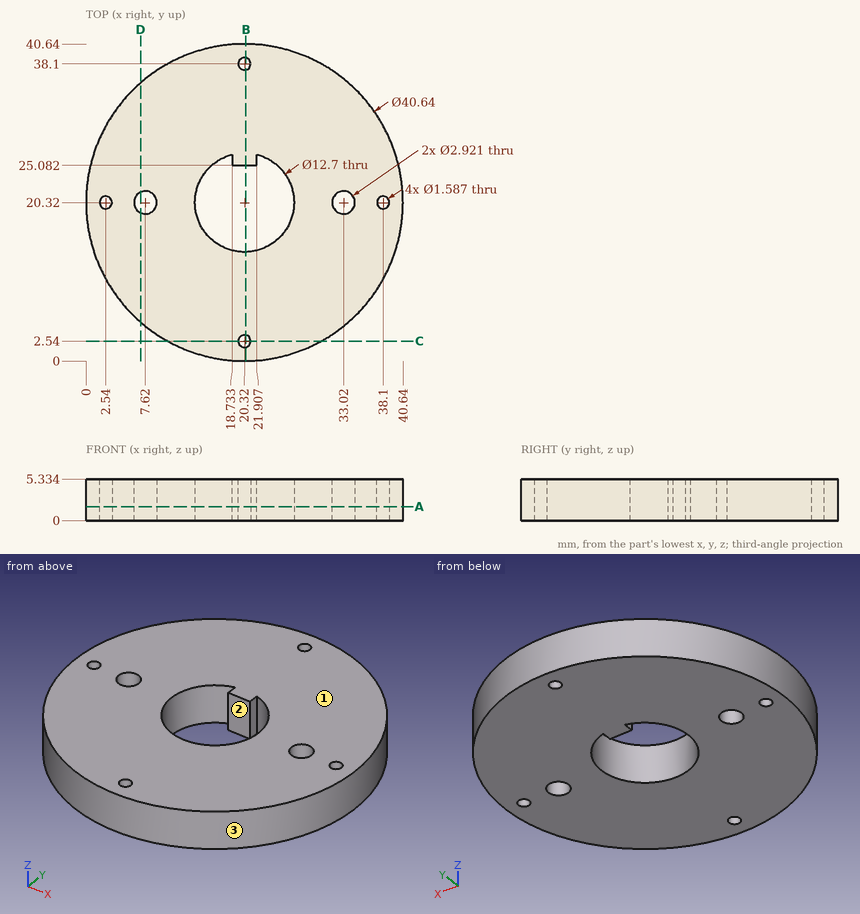
Here's the drawing with two shaded views (mm, measured from the low corner). I have some questions. Coordinates: 2 decimals unless noted, no trailing zeros. Order: outer loops, then holes, each group sorted by start corner. A loop starts at its lowest first (then second) coordinate and runs counter-clockwise, first axis right, second up.
Q1. Will these pins go through, and if not, where does the flat tip stop? pin 1 (1.1 mm diameter, centred on y = 26, z = 4, fed in from +X); pin 2 (1.6 mm diameter, centred on x = 21, z = 2.5, fed in from -Y); pin 3 (1 mm diameter, centred on y = 21, z = 1.5, fed in from +X).
Q2. Suppose I cut it at C-C on y = 2.54. Please give me the cut outline in (x, z) (1 decimal).
Q3. Suppose I cut it at A-A on z = 1.8. Please give me the cut outline in (x, y).
Q4. Thinking about a two-plate mould opening in Y: for the marked faces 1, 2 and 3, which applies, released by +Y, released by -Y, zero draft, split by the parting line, or undercut?
Q5. Please list where these lines run through material, in increasing order: L1, parallel to Y at x = 20.32, z = 3.1; L2, parallel to Y at x = 38.1, z = 2.6 (1 decimal); L3, parallel to X at y = 25, z = 4.45 (1 decimal).
Q6. Suppose I cut it at B-B on x = 20.5. Please give me the cut outline in (y, z) (1 decimal), and give its area (3 significant figures).
Q7. Suppose I cut it at D-D on x = 7. Please give me the cut outline in (y, z) (1 decimal).
Answer:
1. pin 1: stops at x = 39.98
1. pin 2: stops at y = 0
1. pin 3: stops at x = 40.64
2. outline: (10.5, 0) - (19.5, 0) - (19.5, 5.3) - (10.5, 5.3) - close; (21.1, 0) - (30.2, 0) - (30.2, 5.3) - (21.1, 5.3) - close
3. outline: circle Ø40.64 at (20.32, 20.32); hole circle Ø1.59 at (2.54, 20.32); hole circle Ø2.92 at (7.62, 20.32); hole (18.73, 25.08) - (18.73, 26.47) arc R6.35 ccw (long way) to (21.91, 26.47) - (21.91, 25.08) - close; hole circle Ø1.59 at (20.32, 2.54); hole circle Ø1.59 at (20.32, 38.1); hole circle Ø2.92 at (33.02, 20.32); hole circle Ø1.59 at (38.1, 20.32)
4. face 1: zero draft
4. face 2: undercut
4. face 3: split by the parting line
5. L1: y = 0 to 1.75, 3.33 to 13.97, 25.08 to 37.31, 38.89 to 40.64
5. L2: y = 10.5 to 19.5, 21.1 to 30.2
5. L3: x = 0.5 to 16, 24.6 to 40.1
6. outline: (0, 0) - (1.8, 0) - (1.8, 5.3) - (0, 5.3) - close; (3.3, 0) - (14, 0) - (14, 5.3) - (3.3, 5.3) - close; (25.1, 0) - (37.3, 0) - (37.3, 5.3) - (25.1, 5.3) - close; (38.9, 0) - (40.6, 0) - (40.6, 5.3) - (38.9, 5.3) - close
6. area: 141 mm2
7. outline: (5, 0) - (19, 0) - (19, 5.3) - (5, 5.3) - close; (21.6, 0) - (35.7, 0) - (35.7, 5.3) - (21.6, 5.3) - close
